Could you check a few things on this model? Use its own coordinates, in mm. A direction names the side the tool comes from. Coordinates: 2 decimals unless noted, no trailing zeros. Loops run counter-clockwise (first coordinate to the right, second up) from the corner with the lowest first, then second, coordinate; pieces in that order, holes last. Notation, with made-up numbers: M 43.5,47.25 L 70.5,47.25 A17 ccw 70.5,70.25 Z; hole C -7.5,61.25 d6. An arc over 180 degrees is marked long. Return JSON: item names as keys, results as strings. Group by question number.
from build123d import *

# Parameters (mm, degrees)
SKETCH1_R           = 1.6
BOSS_EXTRUDE1_DEPTH = 3
CHAMFER6_SIZE       = 4
CHAMFER5_SIZE       = 0.3
SKETCH8_W           = 8.3
SKETCH8_H           = 3.2
CUT_EXTRUDE1_DEPTH  = 35.336569427


with BuildPart() as part:
    # Sketch1 → Boss-Extrude1 (new body)
    with BuildSketch(Plane.XY):
        with BuildLine():
            Line((-21, 21), (-21, -21))
            Line((-21, -21), (-10, -21))
            Line((-10, -21), (-4, -27))
            Line((-4, -27), (11, -27))
            Line((11, -27), (11.675, -26.325))
            Line((11.675, -26.325), (11.675, -17.331854249))
            Line((11.675, -17.331854249), (3, -8.656854249))
            Line((3, -8.656854249), (3, -5.196152423))
            ThreePointArc((3, -5.196152423), (-6, 0), (3, 5.196152423))
            Line((3, 5.196152423), (3, 8.656854249))
            Line((3, 8.656854249), (11.675, 17.331854249))
            Line((11.675, 17.331854249), (11.675, 26.325))
            Line((11.675, 26.325), (11, 27))
            Line((11, 27), (-4, 27))
            Line((-4, 27), (-10, 21))
            Line((-10, 21), (-21, 21))
        make_face()
        with Locations((-15.5, -15.5)):
            Circle(SKETCH1_R, mode=Mode.SUBTRACT)
        with Locations((-15.5, 15.5)):
            Circle(SKETCH1_R, mode=Mode.SUBTRACT)
    extrude(amount=BOSS_EXTRUDE1_DEPTH)

    # Chamfer6
    chamfer6_edges = [part.edges().sort_by_distance(p)[0] for p in [
        (-21, -21, 1.5),
        (-21, 21, 1.5),
    ]]
    chamfer(chamfer6_edges, length=CHAMFER6_SIZE)

    # Chamfer5
    chamfer5_edges = [part.edges().sort_by_distance(p)[0] for p in [
        (-7, 24, 0),
        (3.5, 27, 0),
        (11.3375, 26.6625, 0),
        (11.675, 21.828427125, 0),
        (7.3375, 12.994354249, 0),
        (3, 6.926503336, 0),
        (-6, 0, 0),
        (3, -6.926503336, 0),
        (7.3375, -12.994354249, 0),
        (11.675, -21.828427125, 0),
        (11.3375, -26.6625, 0),
        (3.5, -27, 0),
        (-7, -24, 0),
        (-13.5, 21, 0),
        (-17.1, -15.5, 0),
        (-17.1, 15.5, 0),
        (-21, 0, 0),
        (-13.5, -21, 0),
        (-19, -19, 0),
        (-19, 19, 0),
    ]]
    chamfer(chamfer5_edges, length=CHAMFER5_SIZE)

    # Sketch8 → Cut-Extrude1 (cut, through all)
    with BuildSketch(Plane.XY.offset(3)):
        with Locations((4.675, 18.6)):
            Rectangle(SKETCH8_W, SKETCH8_H)
        with Locations((4.675, -18.6)):
            Rectangle(SKETCH8_W, SKETCH8_H)
    extrude(amount=-CUT_EXTRUDE1_DEPTH, mode=Mode.SUBTRACT)


solid = part.part
(1) Imagine slicing it at C-C, the plane x = 0. Write out the boundary of the cut face in (y, z).
(2) For faces 4 (the face through (0.525, -19, 2)), 5 (the face through (7.128, 12.994, 0.152)), 6 (the face through (-19, -19, 2)), 7 (the face through (3, -7, 2)), 8 (the face through (-21, 0, 2)), which set-ups out of +Z, -Z, +X, -X, +Y, -Y let a thin tool reach every point of the face, with its end or its side?
(3) We'd pull the mould along X, two halves only. Please class faces 1 (the face through (5, 20.2, 2)), 2 (the face through (-7, 24, 2)), 3 (the face through (-8, 0, 0)): +X half, -X half, draft (parallel to the pull), parting line (faces both ways), or undercut.
(4) Imagine slicing it at A-A, the plane x = -15.5. Write out the boundary of the cut face in (y, z).
(5) Will these pins go through, and if not, where does the flat tip stop? P1, Ø0.8, axis at y = -6.5, z = 2, coming from the +X side; P2, Ø3, axis at x = -15.5, y = -15.5, coming from the +Z side; P3, Ø1.5, axis at x = -10.5, z = 2.5, coming from the -Y side; P4, Ø0.9, axis at y = -18.5, z = 2, coming from the -X side.
(6) Imagine slicing it at B-B, the plane z = 2.25. Write out the boundary of the cut face in (x, y) (3 decimals), then the cut area to 3 significant figures.
(7) Imagine slicing it at D-D, the plane y = -15.5. Write out the boundary of the cut face in (x, z).
(8) If I drill on L1, parallel to Y at x = -15.5, z = 1; L2, parallel to Y at x = 7, z = 0.85; L3, parallel to Y at x = 9.5, z = 0.25, over which ranges is the centre line in solid material (lowest first)? Write a range as [from, to].
Checks:
{
 "1": {"outline": "M -27,0.3 L -26.7,0 L -6.3,0 L -6,0.3 L -6,3 L -27,3 Z; M 6,0.3 L 6.3,0 L 26.7,0 L 27,0.3 L 27,3 L 6,3 Z"},
 "2": {"face 4": "+Z, -Z", "face 5": "-Z, +X", "face 6": "+Z, -Z, -X, -Y", "face 7": "+Z, -Z, +X", "face 8": "+Z, -Z, -X, +Y, -Y"},
 "3": {"face 1": "undercut", "face 2": "-X half", "face 3": "draft"},
 "4": {"outline": "M -21,0.3 L -20.7,0 L -17.4,0 L -17.1,0.3 L -17.1,3 L -21,3 Z; M -13.9,0.3 L -13.6,0 L 13.6,0 L 13.9,0.3 L 13.9,3 L -13.9,3 Z; M 17.1,0.3 L 17.4,0 L 20.7,0 L 21,0.3 L 21,3 L 17.1,3 Z"},
 "5": {"P1": "x = 3", "P2": "through", "P3": "y = -21.25", "P4": "x = -19.95"},
 "6": {"outline": "M -21,-17 L -17,-21 L -10,-21 L -4,-27 L 11,-27 L 11.675,-26.325 L 11.675,-17.332 L 3,-8.657 L 3,-5.196 A6 cw long 3,5.196 L 3,8.657 L 11.675,17.332 L 11.675,26.325 L 11,27 L -4,27 L -10,21 L -17,21 L -21,17 Z; hole C -15.5,-15.5 d3.2; hole C -15.5,15.5 d3.2; hole M 0.525,-20.2 L 8.825,-20.2 L 8.825,-17 L 0.525,-17 Z; hole M 0.525,17 L 8.825,17 L 8.825,20.2 L 0.525,20.2 Z", "area": "1,190 mm²"},
 "7": {"outline": "M -21,0.3 L -20.7,0 L -17.4,0 L -17.1,0.3 L -17.1,3 L -21,3 Z; M -13.9,0.3 L -13.6,0 L 9.42,0 L 9.84,0.3 L 9.84,3 L -13.9,3 Z"},
 "8": {"L1": "[-21, -17.1], [-13.9, 13.9], [17.1, 21]", "L2": "[-27, -20.2], [-17, -12.66], [12.66, 17], [20.2, 27]", "L3": "[-26.95, -15.23], [15.23, 26.95]"}
}
